```python
from build123d import *

# Parameters (mm, degrees)
CHAMFER1_SIZE      = 0.5
SKETCH2_W          = 2
SKETCH2_H          = 2
CUT_EXTRUDE1_DEPTH = 3
SKETCH3_W          = 6
SKETCH3_H          = 5
CUT_EXTRUDE2_DEPTH = 3


with BuildPart() as part:
    # Sketch1 → Revolve1 (revolve)
    with BuildSketch(Plane(origin=(0, 0, 0), x_dir=(0, 0, -1), z_dir=(1, 0, 0)), mode=Mode.PRIVATE) as revolve1_sk:
        Polygon((0.925, 24.1), (0.925, -15), (2.925, -15), (2.925, -2), (1.275, -2), (1.275, 0), (3, 0), (3, 0.753), (2.6, 1.5), (3, 2.247), (3, 3), (1.55, 3), (1.55, 24.1), align=None)
    revolve(revolve1_sk.sketch.rotate(Axis((0, 26.094339623, 0), (0, -1, 0)), 180), axis=Axis((0, 26.094339623, 0), (0, -1, 0)))

    # Chamfer1
    chamfer1_edges = [part.edges().sort_by_distance(p)[0] for p in [
        (0, -2, -2.925),
        (0, -15, -2.925),
    ]]
    chamfer(chamfer1_edges, length=CHAMFER1_SIZE)

    # Sketch2 → Cut-Extrude1 (cut, symmetric)
    with BuildSketch(Plane(origin=(0, 0, 0), x_dir=(0, 0, -1), z_dir=(1, 0, 0))):
        with Locations((-3.25, -3)):
            Rectangle(SKETCH2_W, SKETCH2_H)
        with Locations((3.25, -3)):
            Rectangle(SKETCH2_W, SKETCH2_H)
    extrude(amount=CUT_EXTRUDE1_DEPTH, both=True, mode=Mode.SUBTRACT)

    # Sketch3 → Cut-Extrude2 (cut, symmetric)
    with BuildSketch(Plane(origin=(0, 0, 0), x_dir=(0, 0, -1), z_dir=(1, 0, 0))):
        with Locations((0, 21.6)):
            Rectangle(SKETCH3_W, SKETCH3_H)
    extrude(amount=CUT_EXTRUDE2_DEPTH, both=True, mode=Mode.SUBTRACT)


solid = part.part
```
Could you check a few things on this model? Use its own coordinates, in mm. A direction names the side the tool comes from. Round coordinates to 2 decimals unless told otherwise and drop trailing zeros. Write each loop counter-clockwise with the first axis right and the second up, starting at its lowest first coordinate (ties: lowest second). Pieces come first, ordered by that corner, then holes.
(1) Which directions (+Z, -Z, +X, -X, +Y, -Y) give clear straight access to the entire face, cutting with the end or side of a thin tool? Please do faces 1 (the face through (0, -3, 2.25)), 2 (the face through (-1.1, -2, 1)), 3 (the face through (-2.9, -8.42, -0.38)), 4 (the face through (-0.466, 11.163, 1.478)), 5 (the face through (0, -3, -2.25)).
Findings below:
face 1: +Z, +X, -X
face 2: none
face 3: -Y
face 4: +Y
face 5: -Z, +X, -X
(2) Thinking about a two-plate mould opening in X: for faces 6 (the face through (0.903, 1.811, -0.201)), 7 (the face through (1, -15, -1)), 8 (the face through (-0.383, -0.986, 1.216)), which applies, +X half, -X half, draft (parallel to the pull), parting line (faces both ways), or undercut?
Findings below:
face 6: undercut
face 7: draft
face 8: parting line
(3) Suppose I cut it at C-C on y = 11. Write out the boundary of the cut face in (x, z) (3 decimals), and give its area (3 significant figures).
Findings below:
outline: circle Ø3.1 at (0, 0); hole circle Ø1.85 at (0, 0)
area: 4.86 mm2
(4) For pin 1 (1.1 mm diameter, centred on x = 0, z = 0, fed in from -Y); pin 2 (1.6 mm diameter, centred on x = -0.5, y = -3, fed in from +Z); pin 3 (0.7 mm diameter, centred on x = 0, z = 2.5, fed in from +Y), each with a flat end and sliding along its axis, tell me the tip position at first contact or that it passes through.
Findings below:
pin 1: passes through
pin 2: stops at z = 2.25
pin 3: stops at y = 3
(5) If I drill on probe 1 along X at (y, z) = (4.5, 0) (3 decimals); probe 2 along Y at (x, z) = (1.4, -2.3); probe 3 along Y at (x, z) = (-0.1, 1.95), over which ranges is the centre line in solid material (lowest first)?
Findings below:
probe 1: x = -1.55 to -0.925, 0.925 to 1.55
probe 2: y = -14.73 to -4, 0 to 1.33, 1.67 to 3
probe 3: y = -15 to -2, 0 to 3
(6) Suppose I cut it at D-D on y = -10. Write out the boundary of the cut face in (x, z) (3 decimals).
Findings below:
outline: circle Ø5.85 at (0, 0); hole circle Ø1.85 at (0, 0)
